Here's how the part is built. I have some questions about the finished solid (model axes, mm). Face numbers are marked on the shaded views. A direction names the side the tool comes from. Round coordinates to 2 decimals unless told otherwise and drop trailing zeros. Write each loop counter-clockwise with the first axis right and the second up, starting at its lowest first coordinate (ties: lowest second). Pieces come first, ordered by that corner, then holes. Notation, with made-up numbers: (3.25, 66) -> (54.25, 66) arc R14 cw to (54.25, 93) -> close; hole circle Ø9 at (1, 85.25). An arc over 180 degrees is marked (long way). Put each result on its own line as item: value. Start each with the question number.
1. We'd pull the mould along X, two halves only. Please class the marked faces 4, 5, 6 and 7: +X half, -X half, draft (parallel to the pull), parting line (faces both ways), or undercut.
2. For pin 1 (2 mm diameter, centred on x = 2.5, y = -9, fed in from +Z); pin 2 (2 mm diameter, centred on x = 0, z = -4.5, fed in from -Y); pin 3 (1.5 mm diameter, centred on y = 1.5, z = -0.5, fed in from +X), each with a flat end and sliding along its axis, tell me the tip position at first contact or that it passes through.
3. Suppose I cut it at B-B (x = 0). Please give me the cut outline in (y, z), then the cut area to 3 significant figures.
4. I need wall thicknesses on probe 1 along Y at (x, z) = (0, 5.75); probe 2 along X at (y, z) = (-7.75, -3.75); probe 3 along Y at (x, z) = (0, -3.25). Which ranges of each line are inside material? Lowest first, please. Write a range as from..to.
5. Suppose I cut it at C-C (y = -6.5). Please give me the cut outline in (x, z), then the cut area to 3 significant figures.
6. Suppose I cut it at A-A (z = -0.75). Please give me the cut outline in (x, y).
7. Which directions (+Z, -Z, +X, -X, +Y, -Y) give clear straight access to the entire face, cutting with the end or side of a thin tool? Please do the marked faces 1, 2 and 3.
```python
from build123d import *

# Parameters (mm, degrees)
SKETCH1_R            = 3.6576
SKETCH1_R_2          = 2.3876
BOSS_EXTRUDE1_DEPTH  = 7.62
BOSS_EXTRUDE2_START  = 7.62
BOSS_EXTRUDE2_DEPTH  = 7.62
FILLET1_R            = 1.27
SKETCH5_W            = 2.5622
SKETCH5_H            = 7.62
CUT_EXTRUDE1_DEPTH   = 10.16
FILLET2_R            = 1.27
M3_CLEARANCE_HOLE1_D = 3.6


with BuildPart() as part:
    # Sketch1 → Boss-Extrude1 (new body)
    with BuildSketch(Plane.XY):
        with Locations(Location((0, 0, 0), (0, 0, 180))):
            Circle(SKETCH1_R)
        with Locations(Location((0, 0, 0), (0, 0, 180))):
            Circle(SKETCH1_R_2, mode=Mode.SUBTRACT)
    extrude(amount=BOSS_EXTRUDE1_DEPTH)

    # Sketch4 → Boss-Extrude2 (add)
    with BuildSketch(Plane(origin=(0, 0, 0), x_dir=(-1, 0, 0), z_dir=(0, 0, -1)).offset(BOSS_EXTRUDE2_START)):
        with BuildLine():
            Line((-3.6576, 0), (-3.6576, -15.24))
            Line((-3.6576, -15.24), (3.6576, -15.24))
            Line((3.6576, -15.24), (3.6576, 0))
            ThreePointArc((3.6576, 0), (0, 3.6576), (-3.6576, 0))
        make_face()
    extrude(amount=-BOSS_EXTRUDE2_DEPTH)

    # Fillet1
    fillet1_edges = [part.edges().sort_by_distance(p)[0] for p in [
        (3.6576, -15.24, -3.81),
        (-3.6576, -15.24, -3.81),
    ]]
    fillet(fillet1_edges, radius=FILLET1_R)

    # Sketch5 → Cut-Extrude1 (cut)
    with BuildSketch(Plane.XZ.offset(15.24)):
        with Locations((0, -3.81)):
            Rectangle(SKETCH5_W, SKETCH5_H)
    extrude(amount=-CUT_EXTRUDE1_DEPTH, mode=Mode.SUBTRACT)

    # Fillet2
    # the kernel refuses this fillet: 1.27 mm, written as the material it takes off along each edge
    with BuildSketch(Plane(origin=(1.2811, -15.24, 3.148578796), x_dir=(0, 1, 0), z_dir=(0, 0, -1))) as fillet2_piece_1:
        with BuildLine():
            CenterArc((1.259431519, 1.27), FILLET2_R, 187.396796907, 82.603203093)
            Line((0, 1.1065), (-0.02518863, 1.10323))
            ThreePointArc((-0.02518863, 1.10323), (-0.0254, 0.55325), (-0.0254, 0))
            Line((-0.0254, 0), (0, -0.0254))
            Line((0, -0.0254), (1.259431519, -0.0254))
            Line((1.259431519, -0.0254), (1.259431519, 0))
        make_face()
    extrude(amount=13.917157593, mode=Mode.SUBTRACT)
    with BuildSketch(Plane(origin=(-1.2811, -15.24, -10.768578796), x_dir=(-1, 0, 0), z_dir=(0, 0, 1))) as fillet2_piece_2:
        with BuildLine():
            CenterArc((1.27, -1.259431519), FILLET2_R, 97.396796907, 82.603203093)
            Line((0, -1.259431519), (-0.0254, -1.259431519))
            Line((-0.0254, -1.259431519), (-0.0254, 0))
            Line((-0.0254, 0), (0, 0.0254))
            ThreePointArc((0, 0.0254), (0.55325, 0.0254), (1.10323, 0.02518863))
            Line((1.10323, 0.02518863), (1.1065, 0))
        make_face()
    extrude(amount=13.917157593, mode=Mode.SUBTRACT)

    # M3 Clearance Hole1 (through all)
    with Locations(Plane.XY):
        with Locations((0, 0)):
            Hole(M3_CLEARANCE_HOLE1_D / 2)


solid = part.part
```
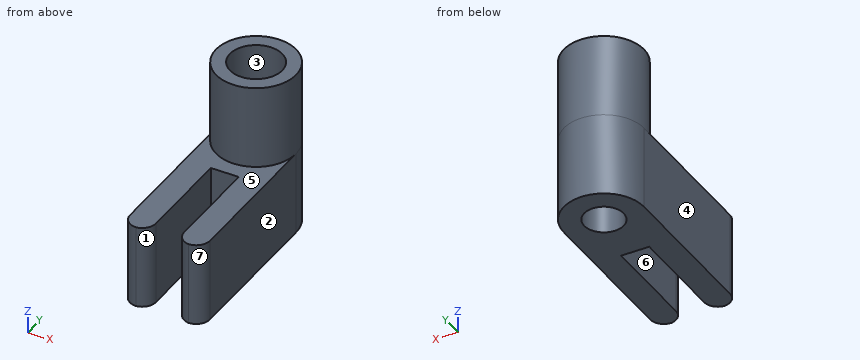
Verdict:
1. face 4: -X half
1. face 5: draft
1. face 6: undercut
1. face 7: +X half
2. pin 1: stops at z = 0
2. pin 2: stops at y = -5.08
2. pin 3: stops at x = 3.58
3. outline: (-5.08, -7.62) -> (-1.8, -7.62) -> (-1.8, 0) -> (-2.39, 0) -> (-2.39, 7.62) -> (-3.66, 7.62) -> (-3.66, 0) -> (-5.08, 0) -> close; (1.8, -7.62) -> (3.66, -7.62) -> (3.66, 7.62) -> (2.39, 7.62) -> (2.39, 0) -> (1.8, 0) -> close
3. area: 58.5 mm^2
4. probe 1: y = -3.66..-2.39, 2.39..3.66
4. probe 2: x = -3.66..-1.28, 1.28..3.66
4. probe 3: y = -5.08..-1.8, 1.8..3.66
5. outline: (-3.66, -7.62) -> (-1.28, -7.62) -> (-1.28, 0) -> (-3.66, 0) -> close; (1.28, -7.62) -> (3.66, -7.62) -> (3.66, 0) -> (1.28, 0) -> close
5. area: 36.2 mm^2
6. outline: (-3.66, -13.97) arc R1.27 ccw to (-2.39, -15.24) arc R1.27 ccw to (-1.28, -13.98) -> (-1.28, -5.08) -> (1.28, -5.08) -> (1.28, -13.98) arc R1.27 ccw to (2.39, -15.24) arc R1.27 ccw to (3.66, -13.97) -> (3.66, 0) arc R3.66 ccw to (-3.66, 0) -> close; hole circle Ø3.6 at (0, 0)
7. face 1: +Z, -Z, -Y
7. face 2: +Z, -Z, +X, +Y, -Y
7. face 3: +Z
